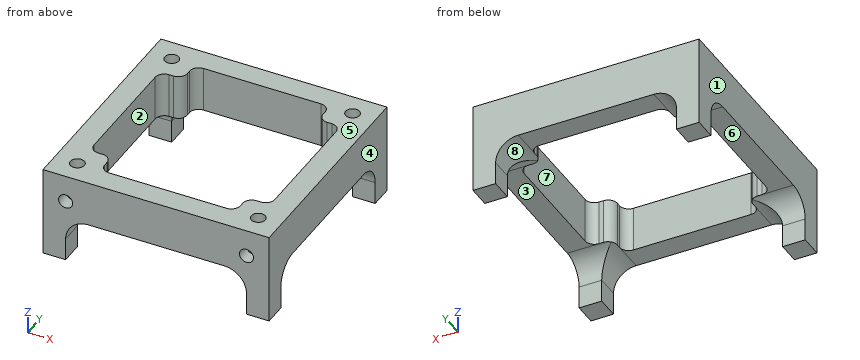
from build123d import *

# Parameters (mm, degrees)
SKETCH152_W     = 50
SKETCH152_H     = 50
PAD026_DEPTH    = 20
POCKET127_DEPTH = 20.001
POCKET128_DEPTH = 50.001
POCKET129_DEPTH = 50.001
SKETCH156_R     = 1.55
POCKET130_DEPTH = 5
SKETCH157_R     = 1.55
POCKET131_DEPTH = 3


with BuildPart() as part:
    # Sketch152 → Pad026 (new body)
    with BuildSketch(Plane.XY):
        Rectangle(SKETCH152_W, SKETCH152_H)
    extrude(amount=PAD026_DEPTH)

    # Sketch153 (on Face6 of Pad026) → Pocket127 (cut, through all)
    with BuildSketch(Plane.XY.offset(20)):
        with BuildLine():
            Line((-18, 15), (-17, 15))
            ThreePointArc((-17, 15), (-15.585786, 15.585786), (-15, 17))
            Line((-15, 17), (-15, 18))
            ThreePointArc((-13, 20), (-14.414214, 19.414214), (-15, 18))
            Line((-13, 20), (13, 20))
            ThreePointArc((15, 18), (14.414214, 19.414214), (13, 20))
            Line((15, 18), (15, 17))
            ThreePointArc((15, 17), (15.585786, 15.585786), (17, 15))
            Line((17, 15), (18, 15))
            ThreePointArc((20, 13), (19.414214, 14.414214), (18, 15))
            Line((20, 13), (20, -13))
            ThreePointArc((18, -15), (19.414214, -14.414214), (20, -13))
            Line((18, -15), (17, -15))
            ThreePointArc((17, -15), (15.585786, -15.585786), (15, -17))
            Line((15, -17), (15, -18))
            ThreePointArc((13, -20), (14.414214, -19.414214), (15, -18))
            Line((13, -20), (-13, -20))
            ThreePointArc((-15, -18), (-14.414214, -19.414214), (-13, -20))
            Line((-15, -18), (-15, -17))
            ThreePointArc((-15, -17), (-15.585786, -15.585786), (-17, -15))
            Line((-17, -15), (-18, -15))
            ThreePointArc((-20, -13), (-19.414214, -14.414214), (-18, -15))
            Line((-20, -13), (-20, 13))
            ThreePointArc((-18, 15), (-19.414214, 14.414214), (-20, 13))
        make_face()
    extrude(amount=-POCKET127_DEPTH, mode=Mode.SUBTRACT)

    # Sketch154 (on Face3 of Pocket127) → Pocket128 (cut, through all)
    with BuildSketch(Plane.YZ.offset(25)):
        with BuildLine():
            Line((-15, 10), (15, 10))
            ThreePointArc((20, 5), (18.535534, 8.535534), (15, 10))
            Line((20, 5), (20, 0))
            Line((20, 0), (-20, 0))
            Line((-20, 0), (-20, 5))
            ThreePointArc((-15, 10), (-18.535534, 8.535534), (-20, 5))
        make_face()
    extrude(amount=-POCKET128_DEPTH, mode=Mode.SUBTRACT)

    # Sketch155 (on Face6 of Pocket127) → Pocket129 (cut, through all)
    with BuildSketch(Plane.XZ.offset(25)):
        with BuildLine():
            Line((-15, 10), (15, 10))
            ThreePointArc((20, 5), (18.535534, 8.535534), (15, 10))
            Line((20, 5), (20, 0))
            Line((20, 0), (-20, 0))
            Line((-20, 0), (-20, 5))
            ThreePointArc((-15, 10), (-18.535534, 8.535534), (-20, 5))
        make_face()
    extrude(amount=-POCKET129_DEPTH, mode=Mode.SUBTRACT)

    # Sketch156 → Pocket130 (cut)
    with BuildSketch(Plane.XY.offset(20)):
        with Locations((-20, 20)):
            Circle(SKETCH156_R)
        with Locations((20, 20)):
            Circle(SKETCH156_R)
        with Locations((20, -20)):
            Circle(SKETCH156_R)
        with Locations((-20, -20)):
            Circle(SKETCH156_R)
    extrude(amount=-POCKET130_DEPTH, mode=Mode.SUBTRACT)

    # Sketch157 (on Face27 of Pocket130) → Pocket131 (cut)
    with BuildSketch(Plane.XZ.offset(25)):
        with Locations((-20, 14)):
            Circle(SKETCH157_R)
        with Locations((20, 14)):
            Circle(SKETCH157_R)
    extrude(amount=-POCKET131_DEPTH, mode=Mode.SUBTRACT)


with BuildPart() as part_1:
    # Body027 placement: moved
    add(part.part.moved(Location((85, 25, 0))))


solid = part_1.part
Model file for the job. Use its own axes, mm. Face numbers are marked on the shaded views. A direction names the side the tool comes from. Round coordinates to 2 decimals unless told otherwise and drop trailing zeros. Loops run counter-clockwise (first coordinate to the right, second up) from the corner with the lowest first, then second, coordinate; pieces in that order, holes last. Notation, with made-up numbers: (17.25, 31) -> (59.25, 31) arc R24 ccw to (59.25, 50) -> close; hole circle Ø5 at (56, 71.5). An arc over 180 degrees is marked (long way). Answer as CSV lines item,"result". Start each with the question number.
1) Probe line 1 along Y through (x, z) = (93.5, 15.25); line 2 along X through (y, z) = (24, 10.75); line 3 along Z through (x, y) = (86, 3.5). List the from-to ranges inside material, lowest first.
2) Tool access for the marked faces 5, 6, 7 and 8: list every direction of +Z, -Z, +X, -X, +Y, -Y with a clear straight run to the whole face (end or side of a thin tool).
3) Mould opens along X. For the marked faces 1, 2, 3 and 4 say: +X half, -X half, draft (parallel to the pull), parting line (faces both ways), or undercut.
4) Slice it at B-B (y = 25). List the corners of the cut face in (x, z), plus the area to 3 significant figures.
5) Slice it at A-A (x = 88). List the corners of the cut face in (y, z), plus the area to 3 significant figures.
6) Pin check, flat tip, straight feed: P1, Ø2, axis at x = 89.5, y = 4, coming from the -Z side. Stop position of the tip, or through.
7) Slice it at C-C (z = 6.5). List the corners of the cut face in (x, y).
Filled in:
1,line 1,"y = 0 to 5, 45 to 50"
1,line 2,"x = 60 to 65, 105 to 110"
1,line 3,"z = 10 to 20"
2,face 5,"+Z, +X, -X, +Y, -Y"
2,face 6,"-Z, +X, -X"
2,face 7,"+Z, -Z"
2,face 8,"-Z, +Y, -Y"
3,face 1,"-X half"
3,face 2,"undercut"
3,face 3,"draft"
3,face 4,"+X half"
4,outline,"(60, 10) -> (65, 10) -> (65, 20) -> (60, 20) -> close; (105, 10) -> (110, 10) -> (110, 20) -> (105, 20) -> close"
4,area,"100 mm2"
5,outline,"(0, 10) -> (5, 10) -> (5, 20) -> (0, 20) -> close; (45, 10) -> (50, 10) -> (50, 20) -> (45, 20) -> close"
5,area,"100 mm2"
6,P1,"stops at z = 10"
7,outline,"(60, 0) -> (65.23, 0) -> (65.23, 5.23) -> (60, 5.23) -> close; (60, 44.77) -> (65.23, 44.77) -> (65.23, 50) -> (60, 50) -> close; (104.77, 0) -> (110, 0) -> (110, 5.23) -> (104.77, 5.23) -> close; (104.77, 44.77) -> (110, 44.77) -> (110, 50) -> (104.77, 50) -> close"
